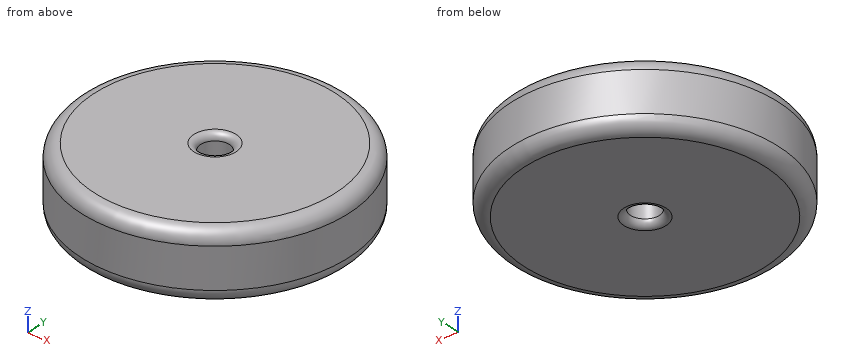
Autodesk Inventor part; units mm, degrees
ref_plane "YZ Plane" through (0, 0, 0) normal (1, 0, 0) x (0, 1, 0)
ref_plane "XZ Plane" through (0, 0, 0) normal (0, 1, 0) x (-1, 0, 0)
ref_plane "XY Plane" through (0, 0, 0) normal (0, 0, 1) x (1, 0, 0)
sketch "Sketch1" plane through (0, 0, 0) normal (0, 0, 1) x (1, 0, 0)
  circle A0 centre (0, 0) radius 2.15
  circle A1 centre (0, 0) radius 20
  dimension "d0" = 4.3
  dimension "d1" = 40
extrude "Extrusion1" add sketch "Sketch1" along normal blind 10
fillet "Fillet1" radius 2 2 edges at (-20, 0, 10) (-20, 0, 0)
fillet "Fillet2" radius 1 2 edges at (-2.15, 0, 10) (-2.15, 0, 0)
properties part number "roller"
Part model, mm, in its own coordinate system. Round coordinates to 2 decimals unless told otherwise and drop trailing zeros. Write each loop counter-clockwise with the first axis right and the second up, starting at its lowest first coordinate (ties: lowest second). Pieces come first, ordered by that corner, then holes. Notation, with made-up numbers: (16.25, -24.75) -> (63.25, -24.75) arc R22 ccw to (63.25, -12.75) -> close; hole circle Ø11 at (42, 59.5). An arc over 180 degrees is marked (long way). Return JSON: item names as keys, results as strings. Group by question number.
Q1. Saw through at C-C on z = 3.25. Write the cut outline in (x, y).
Q2. Probe L1, parallel to Y at x = 0, z = 4; L2, parallel to X at y = -11.5, z = 6.75; L3, parallel to X at y = -10.5, z = 5. List the from-to ranges inside material, lowest first. Write a range as [from, to].
Q3. Pin check, flat tips, straight feed: pin 1 (3 mm diameter, centred on x = 14.5, z = 8, fed in from +Y); pin 2 (5 mm diameter, centred on x = 11, z = 4, fed in from -Y); pin 3 (2 mm diameter, centred on x = 13, y = -4.5, fed in from -Z); pin 4 (5 mm diameter, centred on y = 3.5, z = 1, fed in from -X). Stop position of each tip, or through.
Q4. Saw through at A-A on y = 0. Write the cut outline in (x, z), plus the area to 3 significant figures.
Answer:
{
 "1": {"outline": "circle Ø40 at (0, 0); hole circle Ø4.3 at (0, 0)"},
 "2": {"L1": "[-20, -2.15], [2.15, 20]", "L2": "[-16.36, 16.36]", "L3": "[-17.02, 17.02]"},
 "3": {"pin 1": "y = 15.2", "pin 2": "y = -18.1", "pin 3": "z = 0", "pin 4": "x = -19.96"},
 "4": {"outline": "(-20, 2) arc R2 ccw to (-18, 0) -> (-3.15, 0) arc R1 ccw to (-2.15, 1) -> (-2.15, 9) arc R1 ccw to (-3.15, 10) -> (-18, 10) arc R2 ccw to (-20, 8) -> close; (2.15, 1) arc R1 ccw to (3.15, 0) -> (18, 0) arc R2 ccw to (20, 2) -> (20, 8) arc R2 ccw to (18, 10) -> (3.15, 10) arc R1 ccw to (2.15, 9) -> close", "area": "353 mm2"}
}
